from build123d import *

# Parameters (mm, degrees)
F0_W          = 3
F0_H          = 3
F1_DEPTH      = 1.9
F1_DEPTH_BACK = 1.9


with BuildPart() as f1:
    # F0 (on Right) → F1 (new body, two sides)
    with BuildSketch(Plane.YZ) as f1_sk:
        with BuildLine():
            Line((1.469694, 1.5), (-1.469694, 1.5))
            ThreePointArc((-1.469694, 1.5), (-2.1, 0), (-1.469694, -1.5))
            Line((-1.469694, -1.5), (1.469694, -1.5))
            ThreePointArc((1.469694, -1.5), (1.936021, -0.813524), (2.1, 0))
            ThreePointArc((2.1, 0), (1.936021, 0.813524), (1.469694, 1.5))
        make_face()
        with BuildLine():
            Line((1.469694, -1.5), (-1.469694, -1.5))
            ThreePointArc((-1.469694, -1.5), (0, -2.1), (1.469694, -1.5))
        make_face()
        with BuildLine():
            Line((5.530306, 1.5), (1.469694, 1.5))
            ThreePointArc((1.469694, 1.5), (1.936021, 0.813524), (2.1, 0))
            ThreePointArc((2.1, 0), (1.936021, -0.813524), (1.469694, -1.5))
            Line((1.469694, -1.5), (5.530306, -1.5))
            Line((5.530306, -1.5), (5.530306, 1.5))
        make_face()
        with Locations((7.030306, 0)):
            Rectangle(F0_W, F0_H)
        with BuildLine():
            ThreePointArc((1.469694, 1.5), (0, 2.1), (-1.469694, 1.5))
            Line((-1.469694, 1.5), (1.469694, 1.5))
        make_face()
        with BuildLine():
            ThreePointArc((-1.469694, -1.5), (-2.1, 0), (-1.469694, 1.5))
            Line((-1.469694, 1.5), (-26.469694, 1.5))
            Line((-26.469694, 1.5), (-26.469694, -1.5))
            Line((-26.469694, -1.5), (-1.469694, -1.5))
        make_face()
    extrude(amount=F1_DEPTH)
    extrude(f1_sk.sketch, amount=-F1_DEPTH_BACK)


solid = f1.part
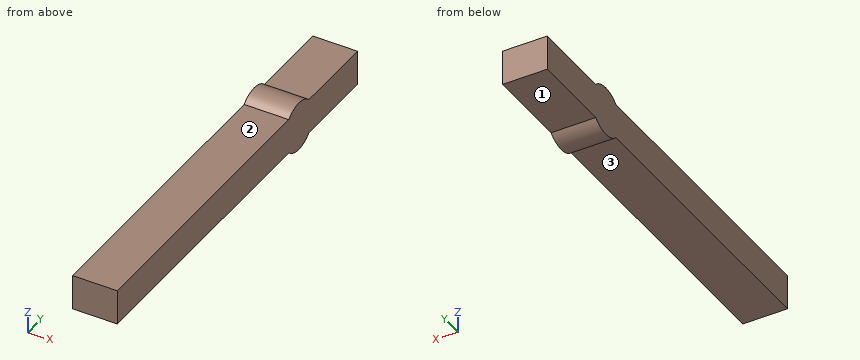
Verification items for the finished model (mm, model axes). Face numbers are marked on the shaded views. A direction names the side the tool comes from. Round coordinates to 2 decimals unless told otherwise and drop trailing zeros. Loops run counter-clockwise (first coordinate to the right, second up) from the corner with the lowest first, then second, coordinate; pieces in that order, holes last. Notation, with made-up numbers: (1, -34.5) - (51, -34.5) arc R16 cw to (51, -16.5) - close; hole circle Ø1 at (-38.75, 14). An arc over 180 degrees is marked (long way). Answer in a Markdown table with one row per item. Add a question column.
Q1. Tool access check on the marked faces 1, 2 and 3. Record the directions out of +Z, -Z, +X, -X, +Y, -Y that give a thin tool (end or side, any length) a straight path to the whole face; none if there is none.
Q2. Section check C-C on y = -1. Enter the section's corners in (x, z), plus the area to 3 significant figures.
Q3. Gauge pin test, flat ends, axial feed: pin 1 (1.1 mm diameter, centred on x = 0, y = -10, fed in from -Z); pin 2 (1.1 mm diameter, centred on x = 0.5, y = 6, fed in from +Z). Record the tip position at first contact, or that the pin passes through.
Q4. Section check B-B on y = -16.5. Enter the section's corners in (x, z), plus the area to 3 significant figures.
Q5. Section check A-A on x = 1.1. Enter the section's corners in (y, z), plus the area to 3 significant figures.
Q6. Material ranges on line 1 (Z direction, x = -0.5, y = -16), recorded low to high.
Found:
| question | item | result |
|---|---|---|
| 1 | face 1 | -Z, +X, -X, +Y |
| 1 | face 2 | +Z, +X, -X, -Y |
| 1 | face 3 | -Z, +X, -X, -Y |
| 2 | outline | (-1.9, -1.85) - (1.9, -1.85) - (1.9, 1.85) - (-1.9, 1.85) - close |
| 2 | area | 14.0 mm² |
| 3 | pin 1 | stops at z = -1.5 |
| 3 | pin 2 | stops at z = 1.5 |
| 4 | outline | (-1.9, -1.5) - (1.9, -1.5) - (1.9, 1.5) - (-1.9, 1.5) - close |
| 4 | area | 11.4 mm² |
| 5 | outline | (-26.47, -1.5) - (-1.47, -1.5) arc R2.1 ccw to (1.47, -1.5) - (8.53, -1.5) - (8.53, 1.5) - (1.47, 1.5) arc R2.1 ccw to (-1.47, 1.5) - (-26.47, 1.5) - close |
| 5 | area | 107 mm² |
| 6 | line 1 | z = -1.5 to 1.5 |
